Print and shaded views of the part. All mm, measured from the part's lowest x, y and z. A direction names the side the tool comes from. Coordinates: 2 decimals unless noted, no trailing zeros. Loops run counter-clockwise (first coordinate to the right, second up) from the corner with the lowest first, then second, coordinate; pieces in that order, holes last.
1) Saw through at D-D, the plane x = 11. Write the cut outline in (y, z), and give its area (3 significant figures).
2) Pin check, flat tips, straight feed: pin 1 Ø5 at (x, y) = (27.5, 18.5) entering from -Z; pin 2 Ø6 at (x, z) = (37.5, 6) entering from +Y; pin 3 Ø4 at (x, z) = (37.5, 69) entering from -Y. Stop position of each tip, or through.
3) Saw through at C-C, the plane y = 81.5. Write the cut outline in (x, z).
4) Which spindle directions (+Z, -Z, +X, -X, +Y, -Y) get a long thin tool onto all of the face, cutting with end or side? Do the marked faces 1 and 2. Say none if no direction does.
5) Saw through at B-B, the plane x = 37.5. Write the cut outline in (y, z).
6) Saw through at A-A, the plane z = 69. Write the cut outline in (x, y), and give its area (3 significant figures).
7) Wall check: line 1 along Y through (x, z) = (37.5, 102.75); line 2 along X through (y, z) = (1, 69); line 3 along Y through (x, z) = (32, 44.5). Give the ranges that are in metal, low to high.
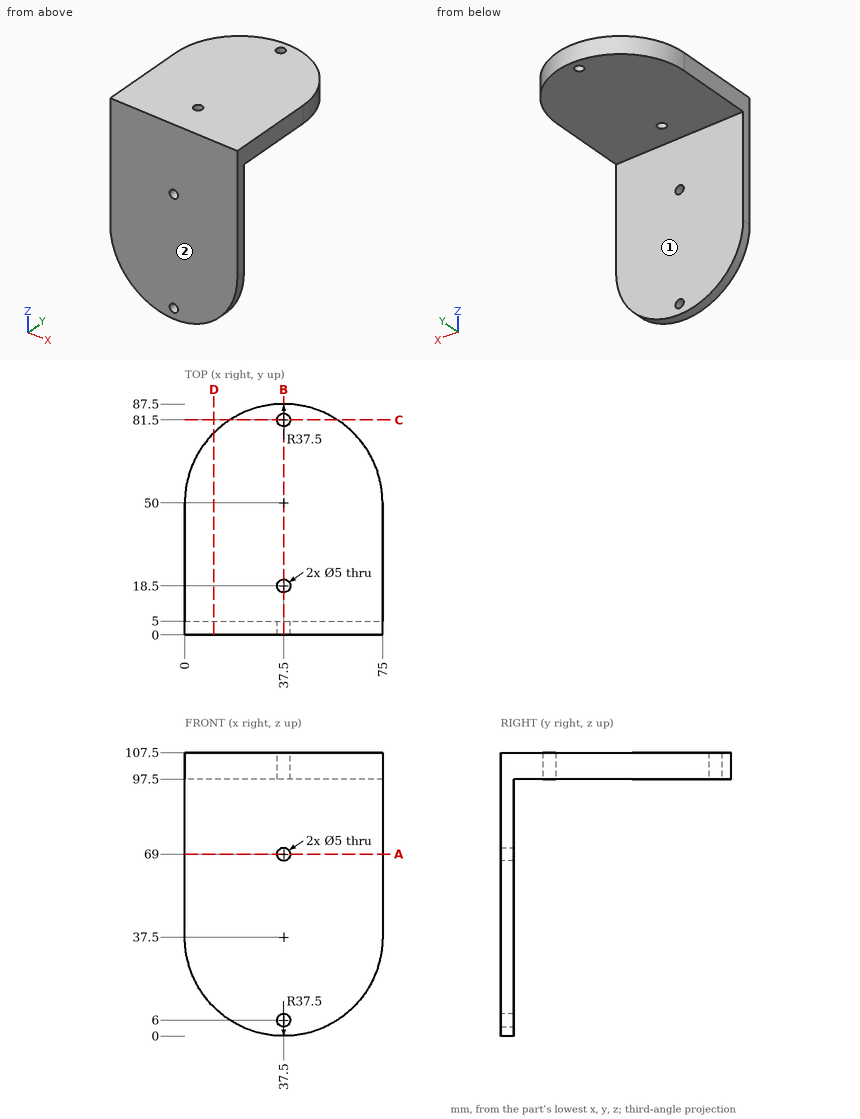
Data:
1. outline: (0, 10.97) - (5, 10.97) - (5, 97.5) - (76.53, 97.5) - (76.53, 107.5) - (0, 107.5) - close
1. area: 1,200 mm2
2. pin 1: stops at z = 97.5
2. pin 2: stops at y = 5
2. pin 3: passes through
3. outline: (17.15, 97.5) - (35, 97.5) - (35, 107.5) - (17.15, 107.5) - close; (40, 97.5) - (57.85, 97.5) - (57.85, 107.5) - (40, 107.5) - close
4. face 1: -Z, +X, -X, +Y
4. face 2: +Z, -Z, +X, -X, -Y
5. outline: (0, 0) - (5, 0) - (5, 3.5) - (0, 3.5) - close; (0, 8.5) - (5, 8.5) - (5, 66.5) - (0, 66.5) - close; (0, 71.5) - (5, 71.5) - (5, 97.5) - (16, 97.5) - (16, 107.5) - (0, 107.5) - close; (21, 97.5) - (79, 97.5) - (79, 107.5) - (21, 107.5) - close; (84, 97.5) - (87.5, 97.5) - (87.5, 107.5) - (84, 107.5) - close
6. outline: (0, 0) - (35, 0) - (35, 5) - (0, 5) - close; (40, 0) - (75, 0) - (75, 5) - (40, 5) - close
6. area: 350 mm2
7. line 1: y = 0 to 16, 21 to 79, 84 to 87.5
7. line 2: x = 0 to 35, 40 to 75
7. line 3: y = 0 to 5
